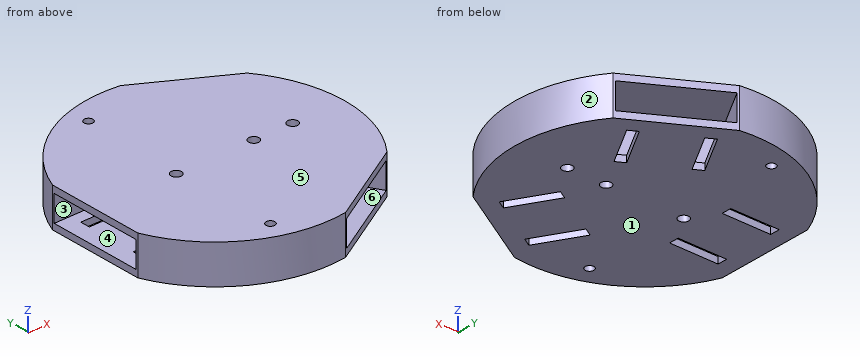
Solid Edge part; units mm, degrees
sketch "Sketch1" plane through (0, 0, 0) normal (0, 0, 1) x (1, 0, 0)
  circle A0 centre (0, 0) radius 40
extrude "Protrusion1" add sketch "Sketch1" along normal blind 12
sketch "Sketch2" plane through (0, 0, 0) normal (0, 0, 1) x (1, 0, 0)
  line L0 (-37.081, 15) -> (-37.081, -15)
extrude "Cutout1" cut sketch "Sketch2" along normal through all material side at (-37.131, 0, 0)
sketch "Sketch3" plane through (-37.081, 0, 6) normal (-1, 0, 0) x (0, -1, 0)
  line L0 (14.4, 4) -> (-14.4, 4)
  line L1 (-14.4, 4) -> (-14.4, -4)
  line L2 (-14.4, -4) -> (14.4, -4)
  line L3 (14.4, -4) -> (14.4, 4)
extrude "Extrusionsausschnitt_5" cut sketch "Sketch3" against normal blind 22
sketch "Sketch4" plane through (-24.581, 0, 2) normal (0, 0, 1) x (0, -1, 0)
  line L0 (-7.75, 7.5) -> (-7.75, -7.5)
  line L1 (-7.75, -7.5) -> (-10.75, -7.5)
  line L2 (-10.75, -7.5) -> (-10.75, 7.5)
  line L3 (-10.75, 7.5) -> (-7.75, 7.5)
extrude "Cutout2" cut sketch "Sketch4" against normal through all
mirror "Mirror1" about plane through (0, 0, 0) normal (0, -1, 0) of "Cutout2"
pattern_circular "Pattern1" count 3 over 360 about axis through (0, 0, 0) along (0, 0, -1) of "Mirror1", "Cutout2", "Extrusionsausschnitt_5", "Cutout1"
hole "Bohrung_3" at (12, 0, 0) direction (0, 0, 1) diameter 3.2 end through all
hole "Hole1" at (24, 0, 0) direction (0, 0, 1) diameter 3.2 end through all
hole "Bohrung_5" at (-12, 0, 0) direction (0, 0, 1) diameter 3.2 end through all
hole "Bohrung_6" at (-11, 32, 0) direction (0, 0, 1) diameter 2.7 end through all
hole "Hole2" at (-11, -32, 0) direction (0, 0, 1) diameter 2.7 end through all
properties material "PVC"
Source: CAD feature listing. Evaluate the final solid. Frame: model axes, mm. Face numbers are marked on the shaded views. A direction names the side the tool comes from. Coordinates: 2 decimals unless noted, no trailing zeros. Write each loop counter-clockwise with the first axis right and the second up, starting at its lowest first coordinate (ties: lowest second). Pieces come first, ordered by that corner, then holes. Notation, with made-up numbers: M -28,61 L -7,61 A21 cw -7,68 Z; hole C -13.75,-20 d3. An arc over 180 degrees is marked long. Answer as a JSON object with one key per item and string values.
1. Cut plane D-D on x = 24. Output: boundary loops of the cut face in (y, z).
Evaluation:
{"outline": "M -28.96,0 L -23.19,0 L -23.19,2 L -28.96,2 Z; M -28.96,10 L -12.77,10 L -12.77,2 L -20.07,2 L -20.07,0 L -1.6,0 L -1.6,12 L -28.96,12 Z; M 1.6,0 L 20.07,0 L 20.07,2 L 12.77,2 L 12.77,10 L 28.96,10 L 28.96,12 L 1.6,12 Z; M 23.19,0 L 28.96,0 L 28.96,2 L 23.19,2 Z"}
2. Access query for the marked faces 5 and 6. Directions: +Z, -Z, +X, -X, +Y, -Y. A direction counts if a zero-diameter tool reaches every point of the face in a straight line with its end or side. Return the directions, or none.
Evaluation:
{"face 5": "+Z, +X, -X, +Y, -Y", "face 6": "none"}
3. Ray query, L1, parallel to X at y = 0, z = 8.75; L2, parallel to Y at x = -11, z = 6.5; L3, parallel to X at y = -1, z = 9.5. Return the intervals inside material, ascending.
Evaluation:
{"L1": "-15.08 to -13.6, -10.4 to 10.4, 13.6 to 22.4, 25.6 to 40", "L2": "-38.46 to -33.35, -30.65 to -1.25, 1.25 to 30.65, 33.35 to 38.46", "L3": "-15.08 to -13.25, -10.75 to 10.75, 13.25 to 22.75, 25.25 to 39.99"}
4. Cut plane A-A on y = 0. Output: boundary loops of the cut face in (x, z).
Evaluation:
{"outline": "M -37.08,0 L -13.6,0 L -13.6,12 L -37.08,12 L -37.08,10 L -15.08,10 L -15.08,2 L -37.08,2 Z; M -10.4,0 L 10.4,0 L 10.4,12 L -10.4,12 Z; M 13.6,0 L 22.4,0 L 22.4,12 L 13.6,12 Z; M 25.6,0 L 40,0 L 40,12 L 25.6,12 Z"}
5. Cut plane B-B on z = 8.5. Output: boundary loops of the cut face in (x, y), plus the area to 3 significant figures.
Evaluation:
{"outline": "M -37.08,-15 A40 ccw 5.55,-39.61 L 6.07,-39.31 L -4.93,-20.26 L 20.01,-5.86 L 31.01,-24.91 L 31.53,-24.61 A40 ccw 31.53,24.61 L 31.01,24.91 L 20.01,5.86 L -4.93,20.26 L 6.07,39.31 L 5.55,39.61 A40 ccw -37.08,15 L -37.08,14.4 L -15.08,14.4 L -15.08,-14.4 L -37.08,-14.4 Z; hole C -12,0 d3.2; hole C -11,-32 d2.7; hole C -11,32 d2.7; hole C 12,0 d3.2; hole C 24,0 d3.2", "area": "2,910 mm^2"}
6. Contact query for flat-ended pins moving along their axis: P1, Ø6.5, axis at y = -4.5, z = 6.5, coming from the -X side; P2, Ø0.6, axis at x = -22.5, z = 1.5, coming from the +Y side; P3, Ø4, axis at y = -10.5, z = 4, coming from the +X side; P4, Ø2.5, axis at x = 24, y = 0, coming from the -Z side. Output: stop coordinate, or through.
Evaluation:
{"P1": "x = -15.08", "P2": "y = 33.27", "P3": "x = 39.09", "P4": "through"}
7. Draft query along Y for the marked faces 1, 2, 3 and 4. Return one class per face: released by +Y, released by -Y, zero draft, split by the parting line, or undercut.
Evaluation:
{"face 1": "zero draft", "face 2": "split by the parting line", "face 3": "undercut", "face 4": "undercut"}
8. Cut plane C-C on y = -27. Output: boundary loops of the cut face in (x, z).
Evaluation:
{"outline": "M -29.51,0 L 3.18,0 L 3.18,2 L -1.04,2 L -1.04,10 L 27.4,10 L 27.4,12 L -29.51,12 Z; M 6.64,0 L 27.4,0 L 27.4,2 L 6.64,2 Z"}
